Check sheet for the modelled part. Datum: model origin and axes. Units: mm. A direction names the side the tool comes from. Give positions to 0.01 mm unless a question says otherwise; leave off trailing zeros. Order: outer loops, then holes, each group sorted by start corner. A loop starts at its lowest first (then second) coordinate and runs counter-clockwise, first axis right, second up. Notation, with made-up numbers: M 68,76.5 L 122,76.5 A30 cw 122,101.5 Z; hole C 19.25,-13.5 d3. An arc over 180 degrees is marked long. Return JSON: item names as keys, results as strings. Group by question number.
from build123d import *

# Parameters (mm, degrees)
F0_W           = 12
F0_H           = 50
F0_R           = 2
F0_W_2         = 0.5
F0_W_3         = 5
F1_DEPTH       = 4
F2_DEPTH       = 8.5
F3_SIZE2       = 3
F3_SIZE        = 4.5
F4_SIZE2       = 3
F4_SIZE        = 4.5
F5_D           = 4
F5_CSINK_D     = 6
F5_CSINK_ANGLE = 90
F6_R           = 0.5


with BuildPart() as f1:
    # F0 (on Front) → F1 (new body)
    with BuildSketch(Plane.XZ):
        Rectangle(F0_W, F0_H)
        with Locations((0, -15)):
            Circle(F0_R, mode=Mode.SUBTRACT)
        with Locations((0, 15)):
            Circle(F0_R, mode=Mode.SUBTRACT)
        with Locations((6.25, 0)):
            Rectangle(F0_W_2, F0_H)
        with Locations((-6.25, 0)):
            Rectangle(F0_W_2, F0_H)
        with Locations((9, 0)):
            Rectangle(F0_W_3, F0_H)
        with Locations((-9, 0)):
            Rectangle(F0_W_3, F0_H)
    extrude(amount=-F1_DEPTH)

    # F0 (on Front) → F2 (join)
    with BuildSketch(Plane.XZ):
        with Locations((-9, 0)):
            Rectangle(F0_W_3, F0_H)
        with Locations((9, 0)):
            Rectangle(F0_W_3, F0_H)
    extrude(amount=-F2_DEPTH)

    # F3
    f3_edges = [f1.edges().sort_by_distance(p)[0] for p in [
        (-11.5, 8.5, 0),
    ]]
    f3_side = f1.faces().sort_by_distance((-11.5, 4.25, 0))[0]
    chamfer(f3_edges, length=F3_SIZE, length2=F3_SIZE2, reference=f3_side)

    # F4
    f4_edges = [f1.edges().sort_by_distance(p)[0] for p in [
        (11.5, 8.5, 0),
    ]]
    f4_side = f1.faces().sort_by_distance((11.5, 4.25, 0))[0]
    chamfer(f4_edges, length=F4_SIZE, length2=F4_SIZE2, reference=f4_side)

    # F5 (through all)
    with Locations(Plane.XZ):
        with Locations((0, 15), (0, -15)):
            CounterSinkHole(F5_D / 2, F5_CSINK_D / 2, counter_sink_angle=F5_CSINK_ANGLE)

    # F6
    f6_edges = [f1.edges().sort_by_distance(p)[0] for p in [
        (10, 6.25, -25),
        (11.5, 4, 0),
        (8.5, 8.5, 0),
        (10, 6.25, 25),
        (7.5, 8.5, -25),
        (6.5, 8.5, 0),
        (7.5, 8.5, 25),
        (-7.5, 8.5, -25),
        (-8.5, 8.5, 0),
        (-6.5, 8.5, 0),
        (-7.5, 8.5, 25),
        (-10, 6.25, 25),
        (-11.5, 4, 0),
        (-10, 6.25, -25),
        (-2, 4, -15),
        (-2, 4, 15),
        (0, 4, -25),
        (6.5, 6.25, -25),
        (-6.5, 6.25, -25),
        (-11.5, 2, -25),
        (11.5, 2, -25),
        (11.5, 2, 25),
        (6.5, 6.25, 25),
        (0, 4, 25),
        (-6.5, 6.25, 25),
        (-11.5, 2, 25),
    ]]
    fillet(f6_edges, radius=F6_R)


solid = f1.part
1) Sectioned sample at A-A on z = 15. Record the boundary of the cut face in (x, y).
2) Sectioned sample at C-C on z = -7. Record the boundary of the cut face in (x, y), then the cut area to 3 significant figures.
3) Depth check by flat-ended pin: P1, Ø4.5, axis at x = 0, z = 15, coming from the -Y side; P2, Ø2, axis at y = 5, z = 2, coming from the +X side; P3, Ø6.5, axis at x = 0.5, z = 0.5, coming from the +Y side. Enter the tip coordinate at first touch or a pass-through.
4) Sectioned sample at D-D on x = -4.5. Record the boundary of the cut face in (y, z), then the cut area to 3 significant figures.
5) Tool access check on faces 4 (the face through (-9.888, 6.147, -24.857)), 5 (the face through (-6.5, 6, 0)). Record the directions out of +Z, -Z, +X, -X, +Y, -Y that give a thin tool (end or side, any length) a straight path to the whole face; none if there is none.
6) Material ranges on line 1 along Z through (x, y) = (0, 1.7); line 2 along X through (y, z) = (3.05, -15); line 3 along X through (y, z) = (6.75, 0), recorded low to high.
7) Sectioned sample at B-B on x = 0. Record the boundary of the cut face in (y, z).
8) Release check for a two-part mould opening along X. For faces 1 (the face through (0.923, 2.232, 13.226)), 2 (the face through (0, 0, 0)), 3 (the face through (-11.5, 2, 0)) record: released by +X, released by -X, zero draft, split by the parting line, or undercut.
Reply:
{
 "1": {"outline": "M -11.5,0 L -3,0 L -2,1 L -2,3.5 A0.5 ccw -2.5,4 L -6.5,4 L -6.5,8 A0.5 ccw -7,8.5 L -8.23,8.5 A0.5 ccw -8.65,8.28 L -11.42,4.13 A0.5 ccw -11.5,3.85 Z; M 2,1 L 3,0 L 11.5,0 L 11.5,3.85 A0.5 ccw 11.42,4.13 L 8.65,8.28 A0.5 ccw 8.23,8.5 L 7,8.5 A0.5 ccw 6.5,8 L 6.5,4 L 2.5,4 A0.5 ccw 2,3.5 Z"},
 "2": {"outline": "M -11.5,0 L 11.5,0 L 11.5,3.85 A0.5 ccw 11.42,4.13 L 8.65,8.28 A0.5 ccw 8.23,8.5 L 7,8.5 A0.5 ccw 6.5,8 L 6.5,4 L -6.5,4 L -6.5,8 A0.5 ccw -7,8.5 L -8.23,8.5 A0.5 ccw -8.65,8.28 L -11.42,4.13 A0.5 ccw -11.5,3.85 Z", "area": "123 mm^2"},
 "3": {"P1": "y = 0.75", "P2": "x = 11.48", "P3": "y = 4"},
 "4": {"outline": "M 0,-25 L 3.5,-25 A0.5 ccw 4,-24.5 L 4,24.5 A0.5 ccw 3.5,25 L 0,25 Z", "area": "200 mm^2"},
 "5": {"face 4": "-Z, -X, +Y", "face 5": "+Z, -Z, +Y"},
 "6": {"line 1": "-25 to -17, -13 to 13, 17 to 25", "line 2": "-11.5 to -2, 2 to 11.5", "line 3": "-9.67 to -6.5, 6.5 to 9.67"},
 "7": {"outline": "M 0,-25 L 3.5,-25 A0.5 ccw 4,-24.5 L 4,-17.5 A0.5 ccw 3.5,-17 L 1,-17 L 0,-18 Z; M 0,-12 L 1,-13 L 3.5,-13 A0.5 ccw 4,-12.5 L 4,12.5 A0.5 ccw 3.5,13 L 1,13 L 0,12 Z; M 0,18 L 1,17 L 3.5,17 A0.5 ccw 4,17.5 L 4,24.5 A0.5 ccw 3.5,25 L 0,25 Z"},
 "8": {"face 1": "undercut", "face 2": "zero draft", "face 3": "released by -X"}
}
